```python
from build123d import *

# Parameters (mm, degrees)
SKETCH_1_R        = 13
EXTRUDE_869_DEPTH = 16
CHAMFER_1_SIZE    = 2


with BuildPart() as part:
    # 草图1 → Extrude 869 (new body)
    with BuildSketch(Plane.XY):
        Polygon((-70, 228), (70, 228), (220, -72), (90, -450), (-90, -450), (-220, -72), align=None)
        with Locations((-140, 0)):
            Circle(SKETCH_1_R, mode=Mode.SUBTRACT)
        with Locations((-60, 0)):
            Circle(SKETCH_1_R, mode=Mode.SUBTRACT)
        with Locations(Location((60, -140, 0), (0, 0, 180))):
            Circle(SKETCH_1_R, mode=Mode.SUBTRACT)
        with Locations(Location((140, -140, 0), (0, 0, 180))):
            Circle(SKETCH_1_R, mode=Mode.SUBTRACT)
        with Locations((-140, -140)):
            Circle(SKETCH_1_R, mode=Mode.SUBTRACT)
        with Locations((-60, -140)):
            Circle(SKETCH_1_R, mode=Mode.SUBTRACT)
        with Locations(Location((60, 0, 0), (0, 0, 180))):
            Circle(SKETCH_1_R, mode=Mode.SUBTRACT)
        with Locations(Location((140, 0, 0), (0, 0, 180))):
            Circle(SKETCH_1_R, mode=Mode.SUBTRACT)
        with Locations((0, -400)):
            Circle(SKETCH_1_R, mode=Mode.SUBTRACT)
        with Locations((0, -240)):
            Circle(SKETCH_1_R, mode=Mode.SUBTRACT)
        with Locations((60, 160)):
            Circle(SKETCH_1_R, mode=Mode.SUBTRACT)
        with Locations((0, -320)):
            Circle(SKETCH_1_R, mode=Mode.SUBTRACT)
        with Locations((-60, 160)):
            Circle(SKETCH_1_R, mode=Mode.SUBTRACT)
        with Locations((56, -240)):
            Circle(SKETCH_1_R, mode=Mode.SUBTRACT)
        with Locations((56, -320)):
            Circle(SKETCH_1_R, mode=Mode.SUBTRACT)
        with Locations((56, -400)):
            Circle(SKETCH_1_R, mode=Mode.SUBTRACT)
        with Locations(Location((-56, -400, 0), (0, 0, 180))):
            Circle(SKETCH_1_R, mode=Mode.SUBTRACT)
        with Locations(Location((-56, -320, 0), (0, 0, 180))):
            Circle(SKETCH_1_R, mode=Mode.SUBTRACT)
        with Locations(Location((-56, -240, 0), (0, 0, 180))):
            Circle(SKETCH_1_R, mode=Mode.SUBTRACT)
    extrude(amount=EXTRUDE_869_DEPTH)

    # 倒角1
    chamfer_1_edges = [part.edges().sort_by_distance(p)[0] for p in [
        (0, -450, 16),
        (155, -261, 16),
        (145, 78, 16),
        (-153, 0, 0),
        (-153, 0, 16),
        (0, 228, 16),
        (-73, 0, 0),
        (-73, 0, 16),
        (73, -140, 0),
        (73, -140, 16),
        (153, -140, 0),
        (153, -140, 16),
        (-153, -140, 0),
        (-153, -140, 16),
        (-73, -140, 0),
        (-73, -140, 16),
        (73, 0, 0),
        (73, 0, 16),
        (-145, 78, 16),
        (153, 0, 0),
        (153, 0, 16),
        (-13, -400, 0),
        (-13, -400, 16),
        (-13, -240, 0),
        (-13, -240, 16),
        (-13, -320, 0),
        (-13, -320, 16),
        (47, 160, 0),
        (47, 160, 16),
        (0, 228, 0),
        (-73, 160, 0),
        (-73, 160, 16),
        (145, 78, 0),
        (43, -240, 0),
        (43, -240, 16),
        (155, -261, 0),
        (43, -320, 0),
        (43, -320, 16),
        (-155, -261, 16),
        (0, -450, 0),
        (43, -400, 0),
        (43, -400, 16),
        (-155, -261, 0),
        (-43, -400, 0),
        (-43, -400, 16),
        (-145, 78, 0),
        (-43, -320, 0),
        (-43, -320, 16),
        (-43, -240, 0),
        (-43, -240, 16),
    ]]
    chamfer(chamfer_1_edges, length=CHAMFER_1_SIZE)


solid = part.part
```
Geometry: final body of the model. Coordinates: model frame, mm. Give positions to 0.01 mm unless a question says otherwise; leave off trailing zeros. Loops run counter-clockwise (first coordinate to the right, second up) from the corner with the lowest first, then second, coordinate; pieces in that order, holes last. Notation, with made-up numbers: (32.5, -20) -> (69.5, -20) arc R17 cw to (69.5, 3) -> close; hole circle Ø1 at (6, 88.5). An arc over 180 degrees is marked (long way). Return JSON: item names as keys, results as strings.
Item 1: Section D-D, the plane x = 140. Output: boundary loops of the cut face in (y, z), plus the area to 3 significant figures.
Filled in:
{"outline": "(-304.62, 2) -> (-298.47, 0) -> (-155, 0) -> (-153, 2) -> (-153, 14) -> (-155, 16) -> (-298.47, 16) -> (-304.62, 14) -> close; (-127, 2) -> (-125, 0) -> (-15, 0) -> (-13, 2) -> (-13, 14) -> (-15, 16) -> (-125, 16) -> (-127, 14) -> close; (13, 2) -> (15, 0) -> (83.53, 0) -> (88, 2) -> (88, 14) -> (83.53, 16) -> (15, 16) -> (13, 14) -> close", "area": "5,410 mm^2"}
Item 2: Line query: line 1 (Y direction, x = 0, z = 4.5); line 2 (Y direction, x = -70, z = 10.75); line 3 (X direction, y = -338, z = 10). Output: solid intervals per line, ascending.
Filled in:
{"line 1": "-450 to -413, -387 to -333, -307 to -253, -227 to 228", "line 2": "-450 to -148.31, -131.69 to -8.31, 8.31 to 151.69, 168.31 to 228", "line 3": "-128.52 to 128.52"}
Item 3: Mould query, pull axis X, two halves, no side actions, for faces 1 (the cylindrical face through (-127.6, 3.9, 7.9)), 2 (the flat face through (143.043, 79.647, 15.014)), 3 (the flat face through (-153.131, -263.316, 15.014)). Classes: released by +X, released by -X, zero draft, split by the parting line, or undercut.
Filled in:
{"face 1": "undercut", "face 2": "released by +X", "face 3": "released by -X"}
Item 4: Pin query (flat end, axial travel): P1, Ø4, axis at y = -207, z = 10.5, coming from the -X side; P2, Ø15.5, axis at x = -60, y = 160, coming from the -Z side; P3, Ø4, axis at x = -93, z = 10, coming from the +Y side; P4, Ø5, axis at y = -173.5, z = 9.5, coming from the -X side. Return the tip coordinate at first contact, or that it passes through.
Filled in:
{"P1": "x = -174.26", "P2": "through", "P3": "y = 186", "P4": "x = -185.95"}
Item 5: Section A-A, the plane x = 0. Count the separate pieces of the cut face and the enclosed holes in it, plus the area to 3 significant figures.
Filled in:
{"separate pieces": "4", "enclosed holes": "0", "area": "9,570 mm^2"}
